The listing builds one solid part. Answer for the finished solid, in the listing's coordinates (mm). Face numbers are marked on the shaded views. A direction names the side the tool comes from. Round coordinates to 2 decimals unless told otherwise and drop trailing zeros. Loops run counter-clockwise (first coordinate to the right, second up) from the corner with the lowest first, then second, coordinate; pieces in that order, holes last. Notation, with made-up numbers: (79, 45) -> (132, 45) arc R22 ccw to (132, 79) -> close; hole circle Ø8 at (26.5, 14). An arc over 180 degrees is marked (long way). Use a Markdown table: item, result. Add a question column.
Q1. Section B-B on y = 58.5 is taken. Give the vertices of the cut face in (x, z), then the cut area to 3 significant figures.
Q2. Section C-C on x = 20.5 is taken. Give the vertices of the cut face in (y, z).
Q3. Section A-A on z = 153.5 is taken. Give the vertices of the cut face in (x, y), then the cut area to 3 significant figures.
Q4. Given pin 1 Ø2 at (y, z) = (-71, 86) entering from -X; pin 2 Ø5 at (x, y) = (58.5, -26) entering from -Z; pin 3 Ø19.5 at (x, y) = (131, -55.5) entering from -Z; pin 4 Ø2 at (x, z) = (25.5, 88.5) entering from +Y, each flat-ended and moving along its own axis, determine where each tip first touches the part or whether it passes through.
Q5. Section D-D on z = 115 is taken. Give the vertices of the cut face in (x, y).
Q6. Which of the six approach directions +Z, -Z, +X, -X, +Y, -Y give full straight-line access (tool end or side, diameter ignored) to the marked faces 4, 5 and 6?
Q7. For a pull along X with two mould halves and no side action, classify the marked faces 1, 2 and 3 as released by +X, released by -X, zero draft, split by the parting line, or undercut.
Q8. Consider line 1 (Y direction, x = 124, z = 17.5); line 2 (Y direction, x = 36.5, z = 50.5); line 3 (X direction, y = -28, z = 67). Determine where each line is inside the solid, lowest interval first.
from build123d import *

# Parameters (mm, degrees)
F1_DEPTH = 143.0895626545
F2_W     = 32.7163190505
F2_H     = 62.8041177988
F5_DEPTH = 25.4


with BuildPart() as f1:
    # F0 (on Top) → F1 (new body)
    with BuildSketch(Plane.XY):
        Polygon((68.2270601392, 72.8508606553), (0, 0), (33.1200025976, -61.8286803365), (126.8782764673, -44.8034033179), align=None)
    extrude(amount=F1_DEPTH)

    # F2 (on face) → F3 (revolve)
    with BuildSketch(Plane(origin=(11.9261231966, -65.6772118101, 0), x_dir=(0.9839099311, 0.1786651828, 0), z_dir=(0.1786651828, -0.9839099311, 0))):
        with Locations((133.190147536, 77.3819759488)):
            Rectangle(F2_W, F2_H)
    revolve(axis=Axis((126.8782764673, -44.8034033179, 77.3819759488), (0, 0, 1)))

    # F4 (on face) → F5 (join)
    with BuildSketch(Plane.XY.offset(143.0895626545)):
        Polygon((126.8782764673, -44.8034033179), (92.4838976122, -51.0489729484), (205.7687044144, -289.458990097), (154.5593430204, -146.4109615539), (113.9569729567, 77.1864652634), (67.0186877251, 145.6461846828), (78.2807342193, 52.6832034748), align=None)
        Polygon((87.7431482077, -25.424644351), (68.2270601392, 0), (92.4838976122, -51.0489729484), (126.8782764673, -44.8034033179), (78.2807342193, 52.6832034748), align=None)
    extrude(amount=F5_DEPTH)


solid = f1.part
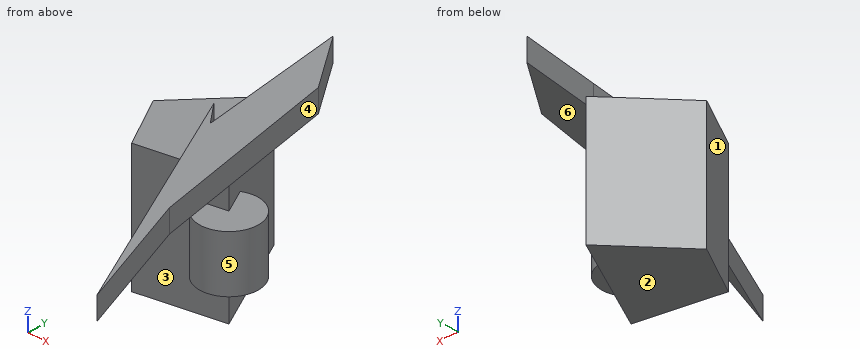
Checked values:
| question | item | result |
|---|---|---|
| 1 | outline | (54.79, 0) -> (75.38, 0) -> (75.38, 143.09) -> (54.79, 143.09) -> close; (77.58, 143.09) -> (117.35, 143.09) -> (117.35, 168.49) -> (77.58, 168.49) -> close |
| 1 | area | 3,960 mm2 |
| 2 | outline | (-38.27, 0) -> (21.89, 0) -> (21.89, 143.09) -> (-38.27, 143.09) -> close |
| 3 | outline | (67.02, 145.65) -> (87.74, -25.42) -> (68.23, 0) -> (205.77, -289.46) -> (154.56, -146.41) -> (113.96, 77.19) -> close |
| 3 | area | 11,100 mm2 |
| 4 | pin 1 | stops at x = 106.01 |
| 4 | pin 2 | stops at z = 0 |
| 4 | pin 3 | stops at z = 45.98 |
| 4 | pin 4 | stops at y = 28.3 |
| 5 | outline | (0, 0) -> (33.12, -61.83) -> (126.88, -44.8) -> (68.23, 72.85) -> close |
| 6 | face 4 | +Z, +X, +Y |
| 6 | face 5 | -Z |
| 6 | face 6 | +X |
| 7 | face 1 | released by -X |
| 7 | face 2 | zero draft |
| 7 | face 3 | undercut |
| 8 | line 1 | y = -45.33 to -39.03 |
| 8 | line 2 | y = -61.21 to 38.97 |
| 8 | line 3 | x = 15 to 154.95 |
